```python
from build123d import *

# Parameters (mm, degrees)
SKETCH1_W           = 106
SKETCH1_H           = 71
BOSS_EXTRUDE1_DEPTH = 30
SKETCH2_W           = 100
SKETCH2_H           = 65
CUT_EXTRUDE1_DEPTH  = 27
SKETCH3_W           = 13
SKETCH3_H           = 7
CUT_EXTRUDE2_DEPTH  = 93.355107755
FILLET1_R           = 2


with BuildPart() as part:
    # Sketch1 → Boss-Extrude1 (new body)
    with BuildSketch(Plane(origin=(0, 0, 0), x_dir=(1, 0, 0), z_dir=(0, 1, 0))):
        with Locations((-1.822129915, 3.859030837)):
            Rectangle(SKETCH1_W, SKETCH1_H)
    extrude(amount=BOSS_EXTRUDE1_DEPTH)

    # Sketch2 → Cut-Extrude1 (cut)
    with BuildSketch(Plane(origin=(0, 30, 0), x_dir=(1, 0, 0), z_dir=(0, 1, 0))):
        with Locations((-1.822129915, 3.859030837)):
            Rectangle(SKETCH2_W, SKETCH2_H)
    extrude(amount=-CUT_EXTRUDE1_DEPTH, mode=Mode.SUBTRACT)

    # Sketch3 → Cut-Extrude2 (cut, through all)
    with BuildSketch(Plane(origin=(0, 0, 28.640969163), x_dir=(-1, 0, 0), z_dir=(0, 0, -1))):
        with Locations((18.322129915, 21.5)):
            Rectangle(SKETCH3_W, SKETCH3_H)
    extrude(amount=-CUT_EXTRUDE2_DEPTH, mode=Mode.SUBTRACT)

    # Fillet1
    fillet1_edges = [part.edges().sort_by_distance(p)[0] for p in [
        (-24.822129915, 25, 30.140969163),
        (-24.822129915, 18, 30.140969163),
        (-11.822129915, 18, 30.140969163),
        (-11.822129915, 25, 30.140969163),
    ]]
    fillet(fillet1_edges, radius=FILLET1_R)


solid = part.part
```
For this review, take the finished solid that the model builds, in its own axes (mm). A direction names the side the tool comes from. Give positions to 0.01 mm unless a question says otherwise; leave off trailing zeros. Order: outer loops, then holes, each group sorted by start corner. A loop starts at its lowest first (then second) coordinate and runs counter-clockwise, first axis right, second up.
1) Wall thickness on line 1 (Z direction, x = -33, y = 24); line 2 (X direction, y = 5.25, z = 14.5); line 3 (Y direction, x = -22, z = -7.5): over which ranges is each line inside the solid? List them lowest first.
2) Insertion check: pin 1 (1 mm diameter, centred on x = -19, z = -7, fed in from +Y). The pin has a flat end and moves straight along its axis. Give the tip position at first contact, or say it passes through.
3) Take a section at D-D (x = -41.5). Give the boundary of the cut face in (y, z).
4) For faces 5 (the face through (-11.822, 21, 30)), 6 (the face through (-3, 0, -4)), 7 (the face through (-3, 17, -36.359)), list the 3-axis set-ups (+Z, -Z, +X, -X, +Y, -Y) from which the entire face can be reached by the end or side of a thin tool; tool diameter is ignored.
5) Take a section at B-B (y = 13.5). Give the boundary of the cut face in (x, z).
6) Take a section at C-C (z = -12). Give the boundary of the cut face in (x, y), then the cut area to 3 significant figures.
7) Take a section at A-A (x = -19). Give the boundary of the cut face in (y, z), then the cut area to 3 significant figures.
8) The part is to be moulded in two halves that separate along Z. For faces 1 (the face through (-51.822, 17, -3)), 2 (the face through (48.178, 17, -3)), 3 (the face through (-24.25, 24.4, 30.16)), 4 (the face through (-3, 15, 31.641)), say which applies: released by +Z, released by -Z, zero draft, split by the parting line, or undercut.
Derived:
1. line 1: z = -39.36 to -36.36, 28.64 to 31.64
1. line 2: x = -54.82 to -51.82, 48.18 to 51.18
1. line 3: y = 0 to 3
2. pin 1: stops at y = 3
3. outline: (0, -39.36) - (30, -39.36) - (30, -36.36) - (3, -36.36) - (3, 28.64) - (30, 28.64) - (30, 31.64) - (0, 31.64) - close
4. face 5: +Z
4. face 6: +Z, -Z, +X, -X, -Y
4. face 7: +Y
5. outline: (-54.82, -39.36) - (51.18, -39.36) - (51.18, 31.64) - (-54.82, 31.64) - close; hole (-51.82, -36.36) - (48.18, -36.36) - (48.18, 28.64) - (-51.82, 28.64) - close
6. outline: (-54.82, 0) - (51.18, 0) - (51.18, 30) - (48.18, 30) - (48.18, 3) - (-51.82, 3) - (-51.82, 30) - (-54.82, 30) - close
6. area: 480 mm2
7. outline: (0, -39.36) - (30, -39.36) - (30, -36.36) - (3, -36.36) - (3, 28.64) - (18, 28.64) - (18, 31.64) - (0, 31.64) - close; (25, 28.64) - (30, 28.64) - (30, 31.64) - (25, 31.64) - close
7. area: 354 mm2
8. face 1: undercut
8. face 2: undercut
8. face 3: zero draft
8. face 4: released by +Z
